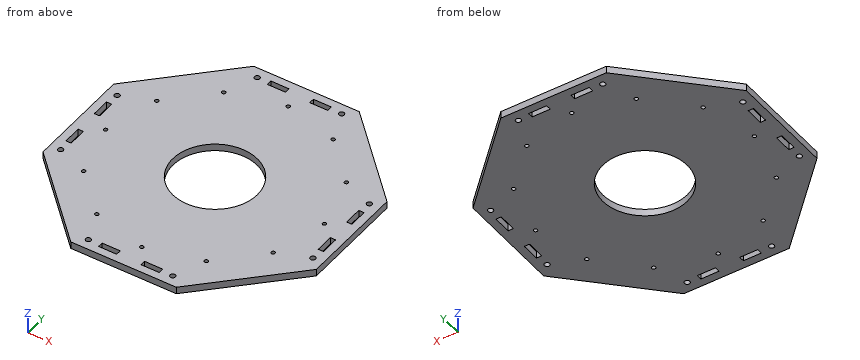
```python
from build123d import *

# Parameters (mm, degrees)
SKETCH1_R           = 109.5
SKETCH1_R_2         = 40
SKETCH1_R_3         = 1.8
BOSS_EXTRUDE1_DEPTH = 6.7
SKETCH4_R           = 109.5
SKETCH4_R_2         = 2.5
SKETCH4_W           = 17.2
SKETCH4_H           = 5
SKETCH4_W_2         = 5
SKETCH4_H_2         = 17.2
BOSS_EXTRUDE2_DEPTH = 6.7


with BuildPart() as part:
    # Sketch1 → Boss-Extrude1 (new body)
    with BuildSketch(Plane.XY):
        Circle(SKETCH1_R)
        Circle(SKETCH1_R_2, mode=Mode.SUBTRACT)
        with Locations((0, 103.7)):
            Circle(SKETCH1_R_3, mode=Mode.SUBTRACT)
        with Locations((51.85, 89.806834372)):
            Circle(SKETCH1_R_3, mode=Mode.SUBTRACT)
        with Locations((89.806834372, 51.85)):
            Circle(SKETCH1_R_3, mode=Mode.SUBTRACT)
        with Locations((103.7, 0)):
            Circle(SKETCH1_R_3, mode=Mode.SUBTRACT)
        with Locations((89.806834372, -51.85)):
            Circle(SKETCH1_R_3, mode=Mode.SUBTRACT)
        with Locations((51.85, -89.806834372)):
            Circle(SKETCH1_R_3, mode=Mode.SUBTRACT)
        with Locations((0, -103.7)):
            Circle(SKETCH1_R_3, mode=Mode.SUBTRACT)
        with Locations((-51.85, -89.806834372)):
            Circle(SKETCH1_R_3, mode=Mode.SUBTRACT)
        with Locations((-89.806834372, -51.85)):
            Circle(SKETCH1_R_3, mode=Mode.SUBTRACT)
        with Locations((-103.7, 0)):
            Circle(SKETCH1_R_3, mode=Mode.SUBTRACT)
        with Locations((-89.806834372, 51.85)):
            Circle(SKETCH1_R_3, mode=Mode.SUBTRACT)
        with Locations((-51.85, 89.806834372)):
            Circle(SKETCH1_R_3, mode=Mode.SUBTRACT)
    extrude(amount=BOSS_EXTRUDE1_DEPTH)

    # Sketch4 → Boss-Extrude2 (add)
    with BuildSketch(Plane.XY):
        Polygon((50, 129.5), (-50, 129.5), (-129.5, 50), (-129.5, -50), (-50, -129.5), (50, -129.5), (129.5, -50), (129.5, 50), align=None)
        Circle(SKETCH4_R, mode=Mode.SUBTRACT)
        with Locations((40, 119.5)):
            Circle(SKETCH4_R_2, mode=Mode.SUBTRACT)
        with Locations(Location((-40, 119.5, 0), (0, 0, 180))):
            Circle(SKETCH4_R_2, mode=Mode.SUBTRACT)
        with Locations(Location((119.5, 40, 0), (0, 0, 180))):
            Circle(SKETCH4_R_2, mode=Mode.SUBTRACT)
        with Locations((119.5, -40)):
            Circle(SKETCH4_R_2, mode=Mode.SUBTRACT)
        with Locations(Location((40, -119.5, 0), (0, 0, 180))):
            Circle(SKETCH4_R_2, mode=Mode.SUBTRACT)
        with Locations((-40, -119.5)):
            Circle(SKETCH4_R_2, mode=Mode.SUBTRACT)
        with Locations(Location((-119.5, -40, 0), (0, 0, 180))):
            Circle(SKETCH4_R_2, mode=Mode.SUBTRACT)
        with Locations((-119.5, 40)):
            Circle(SKETCH4_R_2, mode=Mode.SUBTRACT)
        with Locations((20.1, 119.5)):
            Rectangle(SKETCH4_W, SKETCH4_H, mode=Mode.SUBTRACT)
        with Locations((-20.1, 119.5)):
            Rectangle(SKETCH4_W, SKETCH4_H, mode=Mode.SUBTRACT)
        with Locations((119.5, 20.1)):
            Rectangle(SKETCH4_W_2, SKETCH4_H_2, mode=Mode.SUBTRACT)
        with Locations((119.5, -20.1)):
            Rectangle(SKETCH4_W_2, SKETCH4_H_2, mode=Mode.SUBTRACT)
        with Locations((20.1, -119.5)):
            Rectangle(SKETCH4_W, SKETCH4_H, mode=Mode.SUBTRACT)
        with Locations((-20.1, -119.5)):
            Rectangle(SKETCH4_W, SKETCH4_H, mode=Mode.SUBTRACT)
        with Locations((-119.5, -20.1)):
            Rectangle(SKETCH4_W_2, SKETCH4_H_2, mode=Mode.SUBTRACT)
        with Locations((-119.5, 20.1)):
            Rectangle(SKETCH4_W_2, SKETCH4_H_2, mode=Mode.SUBTRACT)
    extrude(amount=BOSS_EXTRUDE2_DEPTH)


solid = part.part
```
Source: CAD feature listing. Evaluate the final solid. Frame: model axes, mm. Coordinates: 2 decimals unless noted, no trailing zeros. Loops run counter-clockwise (first coordinate to the right, second up) from the corner with the lowest first, then second, coordinate; pieces in that order, holes last. Notation, with made-up numbers: M 25,73 L 69,73 A21 ccw 69,91 Z; hole C 1.5,-7 d9. An arc over 180 degrees is marked long. Use a Markdown table: item, result. Add a question column.
Q1. Section query A-A, the plane x = 17.5. Return loops of the section in (y, z).
Q2. Section query D-D, the plane z = 1.5. State how many separate pieces and enclosed holes the cut face has, and give its area (3 significant figures).
Q3. Material intervals for L1, parallel to Y at x = 25.5, z = 1; L2, parallel to Y at x = -119.5, z = 3.75; L3, parallel to Y at x = -103.7, z = 4, sorted ascending.
Q4. Section query B-B, the plane x = -62. Return loops of the section in (y, z), and give its area (3 significant figures).
Q5. First-contact query: pin 1 (1.5 mm diameter, centred on y = -120.5, z = 3.5, fed in from +X); pin 2 (4 mm diameter, centred on x = -120, z = 2.5, fed in from +Y); pin 3 (4 mm diameter, centred on y = -120, z = 4.5, fed in from +X). Flat tips, straight axial feed; report the tip coordinate or a pass-through.
Q6. Section query C-C, the plane y = -63. Return loops of the section in (x, z).
Result:
| question | item | result |
|---|---|---|
| 1 | outline | M -129.5,0 L -122,0 L -122,6.7 L -129.5,6.7 Z; M -117,0 L -35.97,0 L -35.97,6.7 L -117,6.7 Z; M 35.97,0 L 117,0 L 117,6.7 L 35.97,6.7 Z; M 122,0 L 129.5,0 L 129.5,6.7 L 122,6.7 Z |
| 2 | separate pieces | 1 |
| 2 | enclosed holes | 29 |
| 2 | area | 48,400 mm2 |
| 3 | L1 | y = -129.5 to -122, -117 to -30.82, 30.82 to 117, 122 to 129.5 |
| 3 | L2 | y = -60 to -42.5, -37.5 to -28.7, -11.5 to 11.5, 28.7 to 37.5, 42.5 to 60 |
| 3 | L3 | y = -75.8 to -1.8, 1.8 to 75.8 |
| 4 | outline | M -117.5,0 L 117.5,0 L 117.5,6.7 L -117.5,6.7 Z |
| 4 | area | 1,570 mm2 |
| 5 | pin 1 | stops at x = 59.75 |
| 5 | pin 2 | stops at y = 61.5 |
| 5 | pin 3 | stops at x = 61.5 |
| 6 | outline | M -116.5,0 L 116.5,0 L 116.5,6.7 L -116.5,6.7 Z |
